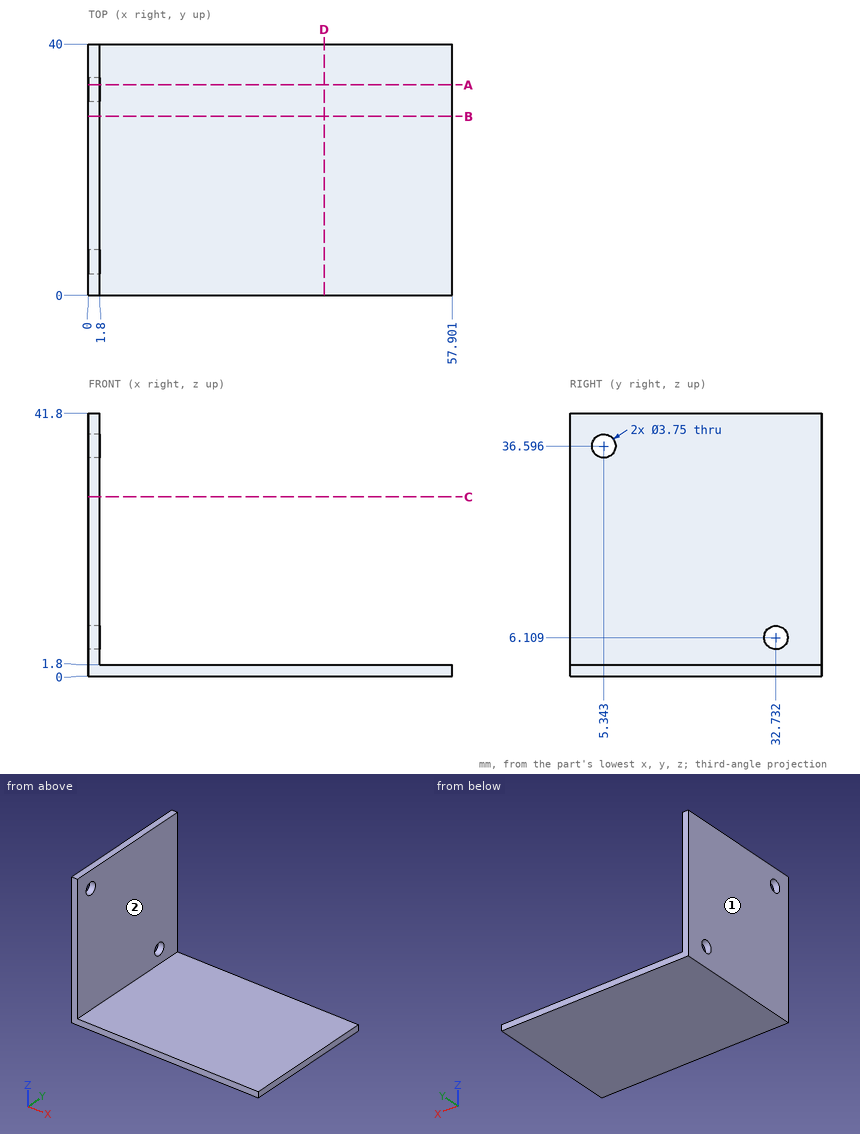
Job drawing, mm, ordinate dimensions from the low corner. One solid piece. A direction names the side the tool comes from. Coordinates: 2 decimals unless noted, no trailing zeros. Order: outer loops, then holes, each group sorted by start corner. A loop starts at its lowest first (then second) coordinate and runs counter-clockwise, first axis right, second up. Notation, with made-up numbers: (14.5, 67) -> (46.5, 67) arc R8 cw to (46.5, 75) -> close; hole circle Ø7 at (56, 60.25). An arc over 180 degrees is marked (long way). Return JSON: item names as keys, results as strings. Group by question number.
Item 1: Tool access for the marked faces 1 and 2: list every direction of +Z, -Z, +X, -X, +Y, -Y with a clear straight run to the whole face (end or side of a thin tool).
Item 2: Wall check: line 1 along X through (y, z) = (36, 18.5). Give the ranges that are in metal, low to high. Write a range as [from, to].
Item 3: Saw through at B-B on y = 28.5. Write the cut outline in (x, z), then the cut area to 3 significant figures.
Item 4: Flat gauge pins, fed straight in: P1, Ø4.5, axis at y = 32.73, z = 6.11, coming from the +X side; P2, Ø3.5, axis at y = 5.34, z = 36.6, coming from the -X side. Where does each tip first touch, or does it go through?
Item 5: Saw through at A-A on y = 33.5. Write the cut outline in (x, z).
Item 6: Saw through at D-D on x = 37.5. Write the cut outline in (y, z).
Item 7: Saw through at C-C on z = 28.5. Write the cut outline in (x, y).
Values found:
{
 "1": {"face 1": "+Z, -Z, -X, +Y, -Y", "face 2": "+Z, +X, +Y, -Y"},
 "2": {"line 1": "x = [0, 1.8]"},
 "3": {"outline": "(0, 0) -> (57.9, 0) -> (57.9, 1.8) -> (1.8, 1.8) -> (1.8, 41.8) -> (0, 41.8) -> close", "area": "176 mm2"},
 "4": {"P1": "stops at x = 1.8", "P2": "passes through"},
 "5": {"outline": "(0, 0) -> (57.9, 0) -> (57.9, 1.8) -> (1.8, 1.8) -> (1.8, 4.4) -> (0, 4.4) -> close; (0, 7.82) -> (1.8, 7.82) -> (1.8, 41.8) -> (0, 41.8) -> close"},
 "6": {"outline": "(0, 0) -> (40, 0) -> (40, 1.8) -> (0, 1.8) -> close"},
 "7": {"outline": "(0, 0) -> (1.8, 0) -> (1.8, 40) -> (0, 40) -> close"}
}
